Source: CAD feature listing. Evaluate the final solid. Frame: model axes, mm. A direction names the side the tool comes from. Give positions to 0.01 mm unless a question says otherwise; leave off trailing zeros. Order: outer loops, then holes, each group sorted by start corner. A loop starts at its lowest first (then second) coordinate and runs counter-clockwise, first axis right, second up.
1) Material intervals for line 1 (Z direction, x = 1.75, y = 1.25); line 2 (X direction, y = -0.5, z = -5.5); line 3 (X direction, y = 2.75, z = -9.25), sorted ascending.
2) Section A-A, the plane x = 0. Return loops of the section in (y, z).
3) First-contact query: P1, Ø5, axis at x = -11, z = -21.5, coming from the -Y side; P2, Ø3, axis at y = -7, z = -9.5, coming from the -X side; P3, Ø1, axis at x = 1, y = 4, coming from the -Z side. Flat tips, straight axial feed; report the tip coordinate or a pass-through.
4) Section C-C, the plane z = -12. Return loops of the section in (x, y), plus the area to 3 significant figures.
5) Access query for faces 1 (the face through (0, 0, -29.2)), 2 (the face through (1.5, -0.07, -27.62)). Directions: +Z, -Z, +X, -X, +Y, -Y. A direction counts if a zero-diameter tool reaches every point of the face in a straight line with its end or side. Return the directions, or none.
```python
from build123d import *

# Parameters (mm, degrees)
CHAMFER1_SIZE = 3


with BuildPart() as part:
    # Sketch1 → Revolve1 (revolve)
    with BuildSketch(Plane(origin=(0, 0, 0), x_dir=(1, 0, 0), z_dir=(0, 1, 0))):
        Polygon((0, 0), (-14, 0), (-14, 26), (-1.5, 26), (-1.5, 29.2), (0, 29.2), align=None)
    revolve(axis=Axis((0, 0, -29.2), (0, 0, 1)))

    # Chamfer1
    chamfer1_edges = [part.edges().sort_by_distance(p)[0] for p in [
        (14, 0, -26),
        (14, 0, 0),
    ]]
    chamfer(chamfer1_edges, length=CHAMFER1_SIZE)


solid = part.part
```
From the geometry:
1. line 1: z = -26 to 0
1. line 2: x = -13.99 to 13.99
1. line 3: x = -13.73 to 13.73
2. outline: (-14, -23) - (-11, -26) - (-1.5, -26) - (-1.5, -29.2) - (1.5, -29.2) - (1.5, -26) - (11, -26) - (14, -23) - (14, -3) - (11, 0) - (-11, 0) - (-14, -3) - close
3. P1: stops at y = -11.12
3. P2: stops at x = -12.87
3. P3: stops at z = -26
4. outline: circle Ø28 at (0, 0)
4. area: 616 mm2
5. face 1: -Z, +X, -X, +Y, -Y
5. face 2: -Z
